Check sheet for the modelled part. Datum: model origin and axes. Units: mm. Face numbers are marked on the shaded views. A direction names the side the tool comes from. Coordinates: 2 decimals unless noted, no trailing zeros. Loops run counter-clockwise (first coordinate to the right, second up) from the corner with the lowest first, then second, coordinate; pieces in that order, holes last.
```python
from build123d import *

# Parameters (mm, degrees)
ESBO_O1_R                = 14
RESSALTO_EXTRUS_O1_DEPTH = 19
ESBO_O2_R                = 4.5
RESSALTO_EXTRUS_O2_DEPTH = 1.5
ESBO_O3_R                = 2.5
RESSALTO_EXTRUS_O3_DEPTH = 10
CORTE_EXTRUS_O1_DEPTH    = 6
CHANFRO2_SIZE            = 0.5
ESBO_O6_R                = 1.75
RESSALTO_EXTRUS_O5_DEPTH = 0.8
FILETE1_R                = 1
RESSALTO_EXTRUS_O6_START = -16
RESSALTO_EXTRUS_O6_DEPTH = 16
RESSALTO_EXTRUS_O7_DEPTH = 12
FILETE2_R                = 0.5
RESSALTO_EXTRUS_O8_DEPTH = 3


with BuildPart() as part:
    # Esboço1 → Ressalto-extrusão1 (new body)
    with BuildSketch(Plane.XY):
        Circle(ESBO_O1_R)
    extrude(amount=RESSALTO_EXTRUS_O1_DEPTH)

    # Esboço2 → Ressalto-extrusão2 (add)
    with BuildSketch(Plane.XY.offset(19)):
        with Locations((0, 8)):
            Circle(ESBO_O2_R)
    extrude(amount=RESSALTO_EXTRUS_O2_DEPTH)

    # Esboço3 → Ressalto-extrusão3 (add)
    with BuildSketch(Plane.XY.offset(19)):
        with Locations((0, 8)):
            Circle(ESBO_O3_R)
    extrude(amount=RESSALTO_EXTRUS_O3_DEPTH)

    # Esboço5 → Corte-extrusão1 (cut)
    with BuildSketch(Plane.XY.offset(29)):
        with BuildLine():
            Line((-1.5, 10.58624067), (-1.5, 5.41375933))
            ThreePointArc((-1.5, 5.41375933), (-2.989755977, 8), (-1.5, 10.58624067))
        make_face()
        with BuildLine():
            Line((1.5, 10.58624067), (1.5, 5.41375933))
            ThreePointArc((1.5, 5.41375933), (2.989755977, 8), (1.5, 10.58624067))
        make_face()
    extrude(amount=-CORTE_EXTRUS_O1_DEPTH, mode=Mode.SUBTRACT)

    # Chanfro2
    chanfro2_edges = [part.edges().sort_by_distance(p)[0] for p in [
        (0, 10.5, 29),
        (0, 5.5, 29),
    ]]
    chamfer(chanfro2_edges, length=CHANFRO2_SIZE)

    # Esboço6 → Ressalto-extrusão5 (add)
    with BuildSketch(Plane.XY.offset(19)):
        with BuildLine():
            Line((17.5, 3.5), (-17.5, 3.5))
            ThreePointArc((-17.5, 3.5), (-21, 0), (-17.5, -3.5))
            Line((-17.5, -3.5), (17.5, -3.5))
            ThreePointArc((17.5, -3.5), (21, 0), (17.5, 3.5))
        make_face()
        with Locations((-17.5, 0)):
            Circle(ESBO_O6_R, mode=Mode.SUBTRACT)
        with Locations((17.5, 0)):
            Circle(ESBO_O6_R, mode=Mode.SUBTRACT)
    extrude(amount=-RESSALTO_EXTRUS_O5_DEPTH)

    # Filete1
    filete1_edges = [part.edges().sort_by_distance(p)[0] for p in [
        (-14, 0, 0),
    ]]
    fillet(filete1_edges, radius=FILETE1_R)

    # Esboço7 → Ressalto-extrusão6 (add)
    with BuildSketch(Plane.XY.offset(19).offset(RESSALTO_EXTRUS_O6_START)):
        with BuildLine():
            Line((7.3, -17), (-7.3, -17))
            Line((-7.3, -17), (-7.3, -11.94612908))
            ThreePointArc((-7.3, -11.94612908), (0, -14), (7.3, -11.94612908))
            Line((7.3, -11.94612908), (7.3, -17))
        make_face()
    extrude(amount=RESSALTO_EXTRUS_O6_DEPTH)

    # Esboço8 → Ressalto-extrusão7 (add)
    with BuildSketch(Plane(origin=(0, 0, 3), x_dir=(-1, 0, 0), z_dir=(0, 0, -1))):
        with BuildLine():
            Line((-7.3, -13.555946275), (-8.8, -12.505634968))
            Line((-8.8, -12.505634968), (-8.8, -10.888526071))
            ThreePointArc((-8.8, -10.888526071), (-8.067349691, -11.441934669), (-7.3, -11.94612908))
            Line((-7.3, -11.94612908), (-7.3, -13.555946275))
        make_face()
        with BuildLine():
            Line((7.3, -13.555946275), (7.3, -11.94612908))
            ThreePointArc((7.3, -11.94612908), (8.067349691, -11.441934669), (8.8, -10.888526071))
            Line((8.8, -10.888526071), (8.8, -12.505634968))
            Line((8.8, -12.505634968), (7.3, -13.555946275))
        make_face()
    extrude(amount=-RESSALTO_EXTRUS_O7_DEPTH)

    # Filete2
    filete2_edges = [part.edges().sort_by_distance(p)[0] for p in [
        (7.3, -14.47306454, 19),
        (-7.3, -15.277973138, 3),
        (8.8, -11.69708052, 3),
        (8.05, -13.030790622, 3),
        (-8.05, -13.030790622, 3),
        (-8.8, -11.69708052, 3),
        (-7.3, -17, 11),
        (7.3, -15.277973138, 3),
        (0, -17, 3),
        (7.3, -17, 11),
        (-7.3, -14.47306454, 19),
        (0, -17, 19),
    ]]
    fillet(filete2_edges, radius=FILETE2_R)

    # Esboço9 → Ressalto-extrusão8 (add)
    with BuildSketch(Plane.XZ.offset(17)):
        with BuildLine():
            Line((-2.75, 17), (2.75, 17))
            ThreePointArc((2.75, 17), (3.4, 16.35), (2.75, 15.7))
            Line((2.75, 15.7), (-2.75, 15.7))
            ThreePointArc((-2.75, 15.7), (-3.4, 16.35), (-2.75, 17))
        make_face()
    extrude(amount=RESSALTO_EXTRUS_O8_DEPTH)


solid = part.part
```
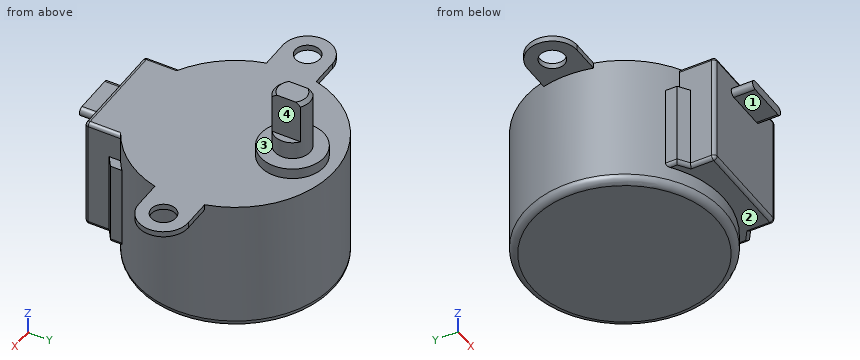
1) Section check C-C on x = -18. Enter the section's corners in (y, z).
Answer sheet:
outline: (-3.46, 18.2) - (-1.68, 18.2) - (-1.68, 19) - (-3.46, 19) - close; (1.68, 18.2) - (3.46, 18.2) - (3.46, 19) - (1.68, 19) - close
2) Depth check by flat-ended pin: pin 1 (8 mm diameter, centred on y = -7.5, z = 26, fed in from +X); pin 2 (3.5 mm diameter, centred on y = -15, z = 13.5, fed in from +X); pin 3 (4 mm diameter, centred on x = 12, z = 15, fed in from -Y); pin 4 (1 mm diameter, centred on x = -1.5, z = 25, fed in from +Y). Enter the tip coordinate at first touch or a pass-through.
Answer sheet:
pin 1: passes through
pin 2: stops at x = 7.74
pin 3: stops at y = -9.8
pin 4: stops at y = 10.29
3) Section check A-A on y = 0. Enter the section's corners in (x, z).
Answer sheet:
outline: (-21, 18.2) - (-19.25, 18.2) - (-19.25, 19) - (-21, 19) - close; (-15.75, 18.2) - (-14, 18.2) - (-14, 1) arc R1 ccw to (-13, 0) - (13, 0) arc R1 ccw to (14, 1) - (14, 18.2) - (15.75, 18.2) - (15.75, 19) - (-15.75, 19) - close; (19.25, 18.2) - (21, 18.2) - (21, 19) - (19.25, 19) - close
4) Set-up check for the marked faces 1, 2, 3 and 4: record each of +Z, -Z, +X, -X, +Y, -Y from which the full face is reachable in a straight line by a thin tool's end or side.
Answer sheet:
face 1: -Z, +X, -X, -Y
face 2: -Z, -Y
face 3: +Z
face 4: +Z, +X, +Y, -Y
5) Section check B-B on z = 5. Enter the section's corners in (x, y), plus the area to 3 significant figures.
Answer sheet:
outline: (-8.8, -12.51) - (-7.3, -13.56) - (-7.3, -16.5) arc R0.5 ccw to (-6.8, -17) - (6.8, -17) arc R0.5 ccw to (7.3, -16.5) - (7.3, -13.56) - (8.8, -12.51) - (8.8, -10.89) arc R14 ccw (long way) to (-8.8, -10.89) - close
area: 674 mm2
6) Section check D-D on x = 15. Enter the section's corners in (y, z).
Answer sheet:
outline: (-3.5, 18.2) - (3.5, 18.2) - (3.5, 19) - (-3.5, 19) - close
7) Scan lines: line 1 (Y direction, x = -17.5, z = 18.65); line 2 (Z direction, x = -3.5, y = -9.5); line 3 (X direction, y = -16.5, z = 11). Record each from-to range of solid material in increasing order.
Answer sheet:
line 1: y = -3.5 to -1.75, 1.75 to 3.5
line 2: z = 0 to 19
line 3: x = -7.3 to 7.3
